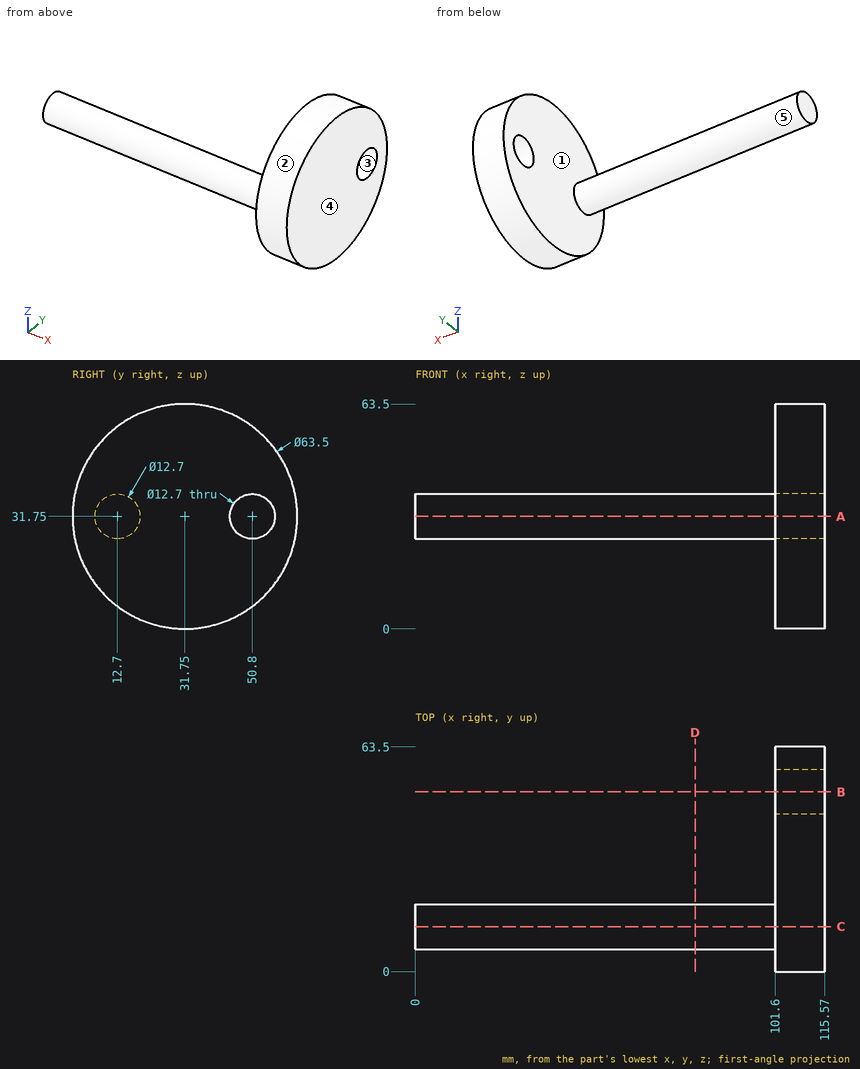
Can you work these out from the drawing? Everything is in mm from the part's minimum corner. A direction names the side the tool comes from. Round coordinates to 2 decimals unless told otherwise and drop trailing zeros. Loops run counter-clockwise (first coordinate to the right, second up) from the corner with the lowest first, then second, coordinate; pieces in that order, holes last. Notation, with made-up numbers: (-16, 79) -> (12, 79) arc R25 cw to (12, 94) -> close; hole circle Ø7 at (9, 19.25). An arc over 180 degrees is marked (long way). Use CSV: the item, a comma, the result in double quotes.
(1) If I drill on probe 1 along Z at (x, y) = (112.75, 50.8); probe 2 along X at (y, z) = (42, 42); probe 3 along Z at (x, y) = (109, 50), over which ranges is the centre line in solid material (lowest first)? Write a range as [from, to].
Return value:
probe 1,"z = [6.35, 25.4], [38.1, 57.15]"
probe 2,"x = [101.6, 115.57]"
probe 3,"z = [5.77, 25.45], [38.05, 57.73]"
(2) For the marked faces 4 and 5, which set-ups out of +Z, -Z, +X, -X, +Y, -Y let a thin tool reach every point of the face, with its end or its side?
Return value:
face 4,"+Z, -Z, +X, +Y, -Y"
face 5,"-X"
(3) Suppose I cut it at B-B on y = 50.8. Write out the boundary of the cut face in (x, z).
Return value:
outline,"(101.6, 6.35) -> (115.57, 6.35) -> (115.57, 25.4) -> (101.6, 25.4) -> close; (101.6, 38.1) -> (115.57, 38.1) -> (115.57, 57.15) -> (101.6, 57.15) -> close"
(4) Suppose I cut it at A-A on z = 31.75. Write out the boundary of the cut face in (x, y).
Return value:
outline,"(0, 6.35) -> (101.6, 6.35) -> (101.6, 0) -> (115.57, 0) -> (115.57, 44.45) -> (101.6, 44.45) -> (101.6, 19.05) -> (0, 19.05) -> close; (101.6, 57.15) -> (115.57, 57.15) -> (115.57, 63.5) -> (101.6, 63.5) -> close"
(5) Will these pins go through, and if not, where does the flat tip stop? pin 1 Ø3 at (y, z) = (48, 17.5) entering from -X; pin 2 Ø2 at (x, z) = (85, 36.5) entering from +Y; pin 3 Ø1 at (x, y) = (85, 9.5) entering from +Z.
Return value:
pin 1,"stops at x = 101.6"
pin 2,"stops at y = 17.82"
pin 3,"stops at z = 37.5"
(6) Suppose I cut it at D-D on x = 79. Write out the boundary of the cut face in (y, z).
Return value:
outline,"circle Ø12.7 at (12.7, 31.75)"
(7) If we mould it in two halves opening along Y, with no side actions, what happens to the marked faces 1, 2 and 3? For each: +Y half, -Y half, draft (parallel to the pull), parting line (faces both ways), or undercut.
Return value:
face 1,"draft"
face 2,"parting line"
face 3,"undercut"
(8) Suppose I cut it at C-C on y = 12.7. Write out the boundary of the cut face in (x, z), plus the area to 3 significant figures.
Return value:
outline,"(0, 25.4) -> (101.6, 25.4) -> (101.6, 6.35) -> (115.57, 6.35) -> (115.57, 57.15) -> (101.6, 57.15) -> (101.6, 38.1) -> (0, 38.1) -> close"
area,"2,000 mm²"
